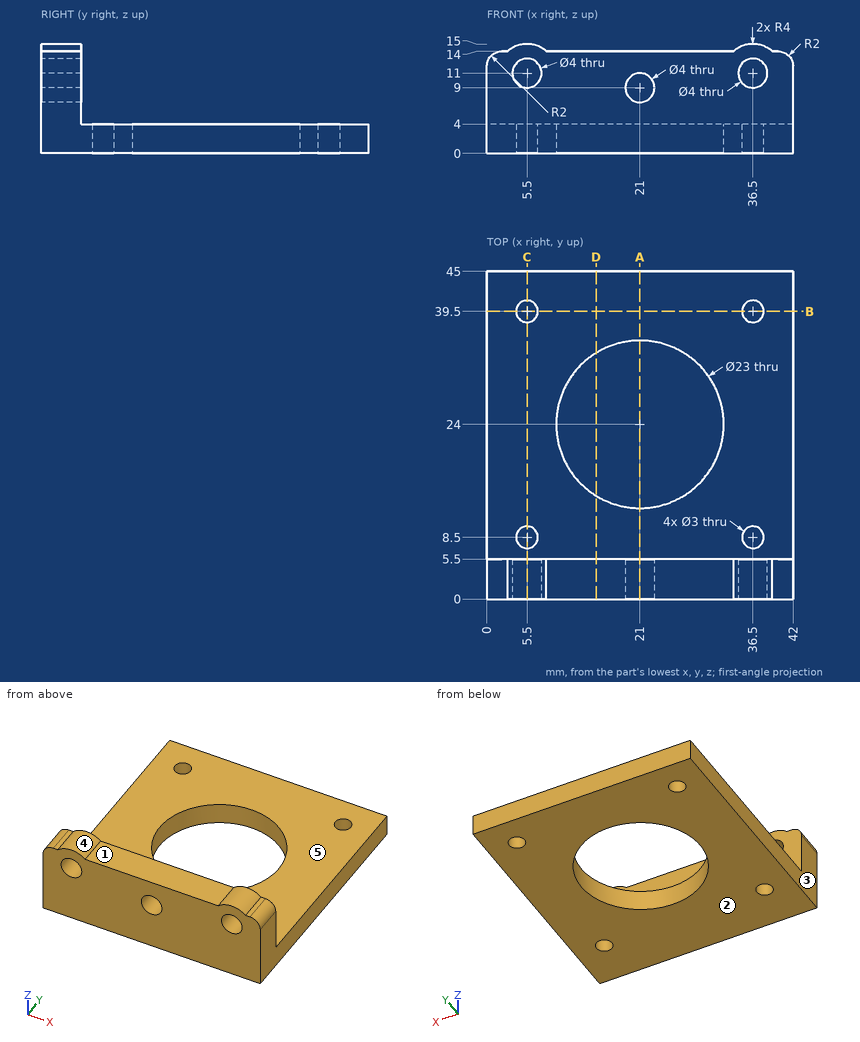
The drawing under review shows one solid part. Ordinate dimensions are in mm from its lowest x, y, z. A direction names the side the tool comes from. Round coordinates to 2 decimals unless told otherwise and drop trailing zeros. Write each loop counter-clockwise with the first axis right and the second up, starting at its lowest first coordinate (ties: lowest second). Pieces come first, ordered by that corner, then holes. Notation, with made-up numbers: (-34.5, 66.5) - (5.5, 66.5) arc R24 cw to (5.5, 89.5) - close; hole circle Ø11 at (-16.5, -24.5). An arc over 180 degrees is marked (long way). One line per question, with ' | ' between items.
Item 1: For the marked faces 4 and 5, list the 3-axis set-ups (+Z, -Z, +X, -X, +Y, -Y) from which the entire face can be reached by the end or side of a thin tool; tool diameter is ignored.
Resolved:
face 4: +Z, +Y, -Y | face 5: +Z, +X, -X, +Y
Item 2: Add section C-C, the plane x = 5.5. Give the boundary of the cut face in (y, z), then the cut area to 4 significant figures.
Resolved:
outline: (0, 0) - (7, 0) - (7, 4) - (5.5, 4) - (5.5, 9) - (0, 9) - close; (0, 13) - (5.5, 13) - (5.5, 15) - (0, 15) - close; (10, 0) - (38, 0) - (38, 4) - (10, 4) - close; (41, 0) - (45, 0) - (45, 4) - (41, 4) - close | area: 194.5 mm2
Item 3: The part is to be moulded in two halves that separate along X. For the marked faces 1, 2 and 3, say which applies: pulls with the +X half, pulls with the -X half, needs draft (parallel to the pull), parting line crosses it, or undercut.
Resolved:
face 1: undercut | face 2: needs draft | face 3: pulls with the -X half
Item 4: For P1, Ø2.5, axis at x = 36.5, y = 8.5, coming from the +Z side; P2, Ø4.5, axis at x = 15.5, y = 2, coming from the +Z side; P3, Ø8, axis at x = 10.5, z = 9, coming from the +Y side; P4, Ø20, axis at x = 15, y = 31.5, coming from the +Z side, all flat-tipped, find the tip position at first contact; note any pin that passes through.
Resolved:
P1: passes through | P2: stops at z = 14 | P3: stops at y = 5.5 | P4: stops at z = 4
Item 5: Add section D-D, the plane x = 15. Give the boundary of the cut face in (y, z).
Resolved:
outline: (0, 0) - (14.19, 0) - (14.19, 4) - (5.5, 4) - (5.5, 14) - (0, 14) - close; (33.81, 0) - (45, 0) - (45, 4) - (33.81, 4) - close
Item 6: To check wall thickness, follow probe 1 along Y at (x, z) = (36.5, 1); probe 2 along Z at (x, y) = (21, 4.15); probe 3 along Z at (x, y) = (21, 40). State the ranges of each line that lie inside material, in increasing order.
Resolved:
probe 1: y = 0 to 7, 10 to 38, 41 to 45 | probe 2: z = 0 to 7, 11 to 14 | probe 3: z = 0 to 4
Item 7: Add section A-A, the plane x = 21. Give the boundary of the cut face in (y, z).
Resolved:
outline: (0, 0) - (12.5, 0) - (12.5, 4) - (5.5, 4) - (5.5, 7) - (0, 7) - close; (0, 11) - (5.5, 11) - (5.5, 14) - (0, 14) - close; (35.5, 0) - (45, 0) - (45, 4) - (35.5, 4) - close
Item 8: Add section B-B, the plane y = 39.5. Give the boundary of the cut face in (x, z).
Resolved:
outline: (0, 0) - (4, 0) - (4, 4) - (0, 4) - close; (7, 0) - (35, 0) - (35, 4) - (7, 4) - close; (38, 0) - (42, 0) - (42, 4) - (38, 4) - close
